Geometry check sheet. Reference: the model listing, model coordinates, mm. Round coordinates to 2 decimals unless told otherwise and drop trailing zeros. Loops run counter-clockwise (first coordinate to the right, second up) from the corner with the lowest first, then second, coordinate; pieces in that order, holes last. Notation, with made-up numbers: (2, 69.5) -> (46, 69.5) arc R19 ccw to (46, 78.5) -> close; hole circle Ø1 at (24, 36). An arc over 180 degrees is marked (long way). Use a Markdown table: item, result. Add a question column.
Q1. Sectioned sample at A-A, the plane y = 10.5. Enter the section's corners in (x, z), then the cut area to 3 significant figures.
Q2. Sectioned sample at B-B, the plane z = -10. Enter the section's corners in (x, y).
Q3. Sectioned sample at C-C, the plane x = 37. Enter the section's corners in (y, z).
Q4. Release check for a two-part mould opening along Y. For faces 1 (the face through (3, -17.97, -0.22)), 2 (the face through (60.84, 18.548, -4.119)), 3 (the face through (5.024, 0.045, -17.999)) record: released by +Y, released by -Y, zero draft, split by the parting line, or undercut.
Q5. Gauge pin test, flat ends, axial feed: P1, Ø2.5, axis at x = 4, y = 0, coming from the -Z side; P2, Ø1.5, axis at x = 45.5, z = 8, coming from the +Y side; P3, Ø1.5, axis at x = 55, y = -13, coming from the +Z side; P4, Ø5, axis at x = 42.5, y = 15, coming from the -Z side. Record the tip position at first contact, or that the pin passes through.
Q6. Material ranges on L1, parallel to X at y = 18, z = 0 (3 decimals); L2, parallel to Y at x = 68, z = 0; L3, parallel to Y at x = 38.5, z = -1.5, recorded low to high.
```python
from build123d import *

# Parameters (mm, degrees)
SKETCH1_W                     = 120
SKETCH1_H                     = 2
M2_5_TAPPED_HOLE1_D           = 2.05
M2_5_TAPPED_HOLE1_ON_FACE_2_D = 2.05
M2_5_TAPPED_HOLE2_D           = 2.05
M2_5_TAPPED_HOLE2_ON_FACE_2_D = 2.05


with BuildPart() as part:
    # Sketch1 → Revolve1 (revolve)
    with BuildSketch(Plane.XY, mode=Mode.PRIVATE) as revolve1_sk:
        with Locations((60, 18)):
            Rectangle(SKETCH1_W, SKETCH1_H)
    revolve(revolve1_sk.sketch.rotate(Axis((-97.700575873, 0, 0), (1, 0, 0)), 90), axis=Axis((-97.700575873, 0, 0), (1, 0, 0)))

    # M2.5 Tapped Hole1 (through all)
    with Locations(Plane(origin=(4, 0, 19), x_dir=(1, 0, 0), z_dir=(0, 0, 1))):
        with Locations((0, 0)):
            Hole(M2_5_TAPPED_HOLE1_D / 2)

    # M2.5 Tapped Hole1 on face 2 (through all)
    with Locations(Plane(origin=(4, -19, 0), x_dir=(0, 0, -1), z_dir=(0, -1, 0))):
        with Locations((0, 0)):
            Hole(M2_5_TAPPED_HOLE1_ON_FACE_2_D / 2)

    # M2.5 Tapped Hole2 (through all)
    with Locations(Plane(origin=(117, 19, 0), x_dir=(0, 0, 1), z_dir=(0, 1, 0))):
        with Locations((0, 0)):
            Hole(M2_5_TAPPED_HOLE2_D / 2)

    # M2.5 Tapped Hole2 on face 2 (through all)
    with Locations(Plane(origin=(117, 0, 19), x_dir=(1, 0, 0), z_dir=(0, 0, 1))):
        with Locations((0, 0)):
            Hole(M2_5_TAPPED_HOLE2_ON_FACE_2_D / 2)


solid = part.part
```
Values:
| question | item | result |
|---|---|---|
| 1 | outline | (0, -15.84) -> (120, -15.84) -> (120, -13.37) -> (0, -13.37) -> close; (0, 13.37) -> (120, 13.37) -> (120, 15.84) -> (0, 15.84) -> close |
| 1 | area | 592 mm^2 |
| 2 | outline | (0, -16.16) -> (120, -16.16) -> (120, -13.75) -> (0, -13.75) -> close; (0, 13.75) -> (120, 13.75) -> (120, 16.16) -> (0, 16.16) -> close |
| 3 | outline | circle Ø38 at (0, 0); hole circle Ø34 at (0, 0) |
| 4 | face 1 | zero draft |
| 4 | face 2 | split by the parting line |
| 4 | face 3 | undercut |
| 5 | P1 | z = -19 |
| 5 | P2 | y = 17.56 |
| 5 | P3 | z = 14.52 |
| 5 | P4 | z = -14.31 |
| 6 | L1 | 0 to 2.975, 5.025 to 115.975, 118.025 to 120 |
| 6 | L2 | -19 to -17, 17 to 19 |
| 6 | L3 | -18.94 to -16.93, 16.93 to 18.94 |
